Build history of the part. All positions in model axes, mm. A direction names the side the tool comes from. Give positions to 0.01 mm unless a question says otherwise; leave off trailing zeros. Order: outer loops, then holes, each group sorted by start corner. A loop starts at its lowest first (then second) coordinate and runs counter-clockwise, first axis right, second up. Notation, with made-up numbers: (-6.5, -36) - (-2.5, -36) arc R9 ccw to (-2.5, -22) - close; hole circle Ø6 at (9, 78.5). An arc over 180 degrees is marked (long way). Answer in a Markdown table with one row per item.
```python
from build123d import *

# Parameters (mm, degrees)
F0_R          = 100.0125
F1_DEPTH      = 31.75
F2_R          = 125
F2_R_2        = 35
F3_DEPTH      = 27.5
F4_R          = 26.9875
F5_DEPTH      = 31.751
F5_DEPTH_BACK = 31.751


with BuildPart() as f1:
    # F0 (on Top) → F1 (new body, symmetric)
    with BuildSketch(Plane.XY):
        Circle(F0_R)
    extrude(amount=F1_DEPTH, both=True)

    # F2 (on Top) → F3 (cut, symmetric)
    with BuildSketch(Plane.XY):
        Circle(F2_R)
        Circle(F2_R_2, mode=Mode.SUBTRACT)
    extrude(amount=F3_DEPTH, both=True, mode=Mode.SUBTRACT)

    # F4 (on Top) → F5 (cut, two sides)
    with BuildSketch(Plane.XY) as f5_sk:
        Circle(F4_R)
    extrude(amount=-F5_DEPTH, mode=Mode.SUBTRACT)
    extrude(f5_sk.sketch, amount=F5_DEPTH_BACK, mode=Mode.SUBTRACT)


solid = f1.part
```
1. Probe line 1 (Z direction, x = -40, y = 52); line 2 (Y direction, x = 0, z = 7); line 3 (Y direction, x = -24.5, z = 26.5) (3 decimals). List the from-to ranges inside material, lowest first.
Check result:
| item | result |
|---|---|
| line 1 | z = -31.75 to -27.5, 27.5 to 31.75 |
| line 2 | y = -35 to -26.99, 26.99 to 35 |
| line 3 | y = -24.995 to -11.317, 11.317 to 24.995 |
2. Cut at D-D on x = -86. Write the cut outline in (y, z), and give its area (3 significant figures).
Check result:
| item | result |
|---|---|
| outline | (-51.05, -31.75) - (51.05, -31.75) - (51.05, -27.5) - (-51.05, -27.5) - close; (-51.05, 27.5) - (51.05, 27.5) - (51.05, 31.75) - (-51.05, 31.75) - close |
| area | 868 mm² |
3. Cut at A-A on y = 0. Write the cut outline in (x, z), and give its area (3 significant figures).
Check result:
| item | result |
|---|---|
| outline | (-100.01, -31.75) - (-26.99, -31.75) - (-26.99, 31.75) - (-100.01, 31.75) - (-100.01, 27.5) - (-35, 27.5) - (-35, -27.5) - (-100.01, -27.5) - close; (26.99, -31.75) - (100.01, -31.75) - (100.01, -27.5) - (35, -27.5) - (35, 27.5) - (100.01, 27.5) - (100.01, 31.75) - (26.99, 31.75) - close |
| area | 2,120 mm² |
4. Which spindle directions (+Z, -Z, +X, -X, +Y, -Y) get a long thin tool onto all of the face, cutting with end or side? Do faces 4 (the face through (-21.681, -97.634, -29.595)), 5 (the face through (43, 1, -27.5)). Say none if no direction does.
Check result:
| item | result |
|---|---|
| face 4 | +Z, -Z |
| face 5 | none |
5. Cut at C-C on z = -21.5. Write the cut outline in (x, y) (1 decimal).
Check result:
| item | result |
|---|---|
| outline | circle Ø70 at (0, 0); hole circle Ø54 at (0, 0) |
6. Drop flat-ended pins along their axis: P1, Ø3, axis at y = 32, z = 21.5, coming from the -X side; P2, Ø5, axis at y = -23, z = -6.5, coming from the -X side; P3, Ø8, axis at x = 19.5, z = 2, coming from the +Y side. Give the stop position or say it passes through.
Check result:
| item | result |
|---|---|
| P1 | stops at x = -17.17 |
| P2 | stops at x = -28.37 |
| P3 | stops at y = 31.38 |
7. Two-plate mould, pull along X, no slides. Class faces 1 (the face through (-19.89, 18.24, 0.44)), 2 (the face through (-28, -21, 0)), 3 (the face through (43, 1, 27.5)): +X half, -X half, draft (parallel to the pull), parting line (faces both ways), or undercut.
Check result:
| item | result |
|---|---|
| face 1 | undercut |
| face 2 | parting line |
| face 3 | draft |
